Work out the finished part from the listing and answer in its coordinate system (mm). Face numbers are marked on the shaded views. A direction names the side the tool comes from. Round coordinates to 2 decimals unless told otherwise and drop trailing zeros. Write each loop counter-clockwise with the first axis right and the second up, starting at its lowest first coordinate (ties: lowest second). Pieces come first, ordered by that corner, then holes.
1. Straight lines are drawn through the part: probe 1 along X at (y, z) = (0, 9.5); probe 2 along X at (y, z) = (0, 13.5); probe 3 along Z at (x, y) = (2.5, 10.5). For each, find the intervals that lie inside material, in ascending order.
2. Find section C-C (y = -6). Write down the section's boundary in (x, z), and give its area (3 significant figures).
3. A tool of negligible diameter and unlimited length cuts with its end or side. For the marked faces 4, 5 and 6, from which of +Z, -Z, +X, -X, +Y, -Y can it reach the whole face along a straight path? Write none if from no direction.
4. Determine the mould class of the marked faces 1, 2 and 3 for opening direction Y: pulls with the +Y half, pulls with the -Y half, needs draft (parallel to the pull), parting line crosses it, or undercut.
5. Find section D-D (y = -9). Write down the section's boundary in (x, z).
6. Find section A-A (y = 0). Write down the section's boundary in (x, z), and give its area (3 significant figures).
7. Flat-ended cylindrical pins translate along their axes: pin 1 Ø1.5 at (x, z) = (-7, 5.5) entering from +Y; pin 2 Ø4 at (x, z) = (5.5, 6) entering from -Y; pin 3 Ø1 at (x, z) = (1, 5) entering from +Y. Find the tip coordinate at first contact, or state that the pin passes through.
8. Find section B-B (z = 11.75). Write down the section's boundary in (x, y), and give its area (3 significant figures).
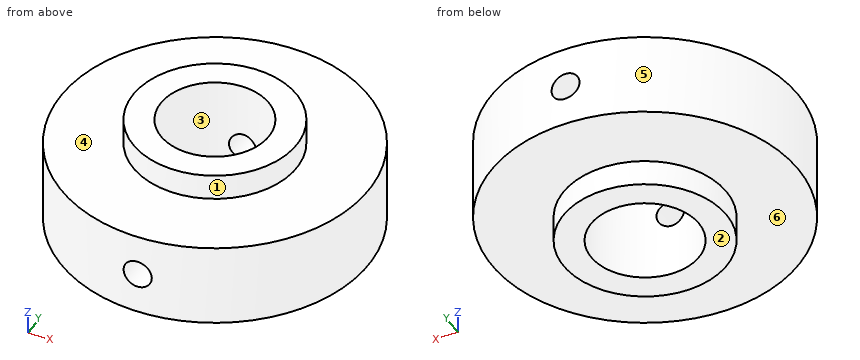
```python
from build123d import *

# Parameters (mm, degrees)
SKETCH1_W          = 2.15
SKETCH1_H          = 2.03
SKETCH2_R          = 1.0922
CUT_EXTRUDE1_DEPTH = 24.876


with BuildPart() as part:
    # Sketch1 → Revolve1 (revolve)
    with BuildSketch(Plane(origin=(0, 0, 0), x_dir=(1, 0, 0), z_dir=(0, 1, 0))):
        with Locations((-2.995601826, -13.170436757)):
            Rectangle(SKETCH1_W, SKETCH1_H)
        Polygon((-4.070601826, -12.155436757), (-1.920601826, -12.155436757), (-1.920601826, -3.573436757), (-4.070601826, -3.573436757), (-4.070601826, -5.605436757), align=None)
        Polygon((-5.107903637, -12.155436757), (-4.070601826, -12.155436757), (-4.070601826, -5.605436757), (-9.658601826, -5.605436757), (-9.658601826, -12.155436757), align=None)
    revolve(axis=Axis((2.279398174, 0, -19.129935757), (0, 0, 1)))

    # Sketch2 → Cut-Extrude1 (cut, through all)
    with BuildSketch(Plane(origin=(0, 11.938, 0), x_dir=(1, 0, 0), z_dir=(0, 1, 0))):
        with Locations((2.369164509, -8.88650333)):
            Circle(SKETCH2_R)
    extrude(amount=-CUT_EXTRUDE1_DEPTH, mode=Mode.SUBTRACT)


solid = part.part
```
Worked answers:
1. probe 1: x = -9.66 to -1.92, 6.48 to 14.22
1. probe 2: x = -4.07 to -1.92, 6.48 to 8.63
1. probe 3: z = 5.61 to 7.8, 9.97 to 12.16
2. outline: (-8.04, 5.61) - (0.2, 5.61) - (0.2, 3.57) - (4.36, 3.57) - (4.36, 5.61) - (12.6, 5.61) - (12.6, 12.16) - (4.36, 12.16) - (4.36, 14.19) - (0.2, 14.19) - (0.2, 12.16) - (-8.04, 12.16) - close; hole circle Ø2.18 at (2.37, 8.89)
2. area: 148 mm2
3. face 4: +Z
3. face 5: +Z, -Z
3. face 6: -Z
4. face 1: parting line crosses it
4. face 2: needs draft
4. face 3: undercut
5. outline: (-5.56, 5.61) - (10.12, 5.61) - (10.12, 12.16) - (-5.56, 12.16) - close; hole circle Ø2.18 at (2.37, 8.89)
6. outline: (-9.66, 5.61) - (-4.07, 5.61) - (-4.07, 3.57) - (-1.92, 3.57) - (-1.92, 14.19) - (-4.07, 14.19) - (-4.07, 12.16) - (-9.66, 12.16) - close; (6.48, 3.57) - (8.63, 3.57) - (8.63, 5.61) - (14.22, 5.61) - (14.22, 12.16) - (8.63, 12.16) - (8.63, 14.19) - (6.48, 14.19) - close
6. area: 119 mm2
7. pin 1: stops at y = 8.34
7. pin 2: stops at y = -11.88
7. pin 3: stops at y = 6.3
8. outline: circle Ø23.88 at (2.28, 0); hole circle Ø8.4 at (2.28, 0)
8. area: 392 mm2
